Can you work these out from the model? Positions are in its coordinate system, mm. A direction names the side the tool comes from. Round coordinates to 2 decimals unless told otherwise and drop trailing zeros. Write each loop counter-clockwise with the first axis right and the second up, starting at its lowest first coordinate (ties: lowest second). Pieces come first, ordered by that corner, then holes. Notation, with made-up numbers: M -27,59.25 L 17,59.25 A18 cw 17,79.25 Z; hole C 53,67 d5. An arc over 180 degrees is marked long. Answer as a JSON object with one key per item and string values. Group by question number.
1) If we mould it in two halves opening along Z, with no side actions, what happens to faces 1 (the cylindrical face through (-22.316, 9.268, 5.276)), 2 (the flat face through (-15, 17, 4)), 3 (the cylindrical face through (11.353, 19.746, 14.757)), 4 (the cylindrical face through (-22.316, 9.268, 15.276))? For each: +Z half, -Z half, draft (parallel to the pull), parting line (faces both ways), or undercut.
2) Please list where these lines run through material, in increasing order: L1, parallel to X at y = 9.5, z = 3.5; L2, parallel to Y at x = -3.5, z = 17.75; L3, parallel to X at y = 1, z = 11.75. Write a range as [from, to].
3) I'm going to push flat-ended pins straight in: pin 1 Ø4 at (x, z) = (24.5, 9.5) entering from +Y; pin 2 Ø1.5 at (x, z) = (8.5, 3.5) entering from +Y; pin 3 Ø1.5 at (y, z) = (15.5, 15.5) entering from +X; pin 4 Ø3 at (x, z) = (24.315, 15.2) entering from +Y (3 decimals). Where does each tip first touch, or does it pass through?
4) Suppose I cut it at A-A, the plane y = -14. Write out the boundary of the cut face in (x, z), and give its area (3 significant figures).
5) Suppose I cut it at B-B, the plane x = -7.5. Write out the boundary of the cut face in (y, z).
6) On a 3-axis mill with a long thin cutter (end or side, diameter ignored), from which of +Z, -Z, +X, -X, +Y, -Y can I reach the whole of each face in a straight line? I mean faces 5 (the flat face through (-20.15, 13, 10)), 6 (the flat face through (-15, 17, 17)), 7 (the flat face through (20.15, 13, 10)), 8 (the flat face through (27, 9, 3)), 9 (the flat face through (-18, 15.5, 10)). Say none if no direction works.
from build123d import *

# Parameters (mm, degrees)
EXTRUDE_1_DEPTH        = 20
FILLET_1_R             = 1
CUT_EXTRUDE_1_DEPTH    = 20
SKETCH_3_W             = 51.867663345
SKETCH_3_H             = 35.261757523
CUT_EXTRUDE_2_DEPTH    = 3
SKETCH_4_R             = 6
EXTRUDE_2_DEPTH        = 1
SKETCH_5_R             = 5
EXTRUDE_3_DEPTH        = 0.5
SKETCH_6_R             = 1
EXTRUDE_4_DEPTH        = 4
HOLE_WIZARD_M3_1_D     = 2.5
HOLE_WIZARD_M3_1_DEPTH = 7.5
HOLE_WIZARD_M3_1_TIP   = 0.751075774


with BuildPart() as part:
    # 草图1 → 凸台-拉伸1 (new body)
    with BuildSketch(Plane.XY):
        Polygon((20.15, 8), (27, 8), (27, 10.5), (20.15, 10.5), (20.15, 18.5), (-20.15, 18.5), (-20.15, 10.5), (-27, 10.5), (-27, 8), (-20.15, 8), (-20.15, -19), (20.15, -19), align=None)
    extrude(amount=EXTRUDE_1_DEPTH)

    # 圆角1
    fillet_1_edges = [part.edges().sort_by_distance(p)[0] for p in [
        (-27, 9.25, 20),
        (20.15, 14.5, 0),
        (27, 9.25, 0),
        (20.15, -5.5, 0),
        (0, -19, 0),
        (-20.15, -5.5, 0),
        (-27, 9.25, 0),
        (-20.15, 14.5, 0),
        (-20.15, -5.5, 20),
        (0, -19, 20),
        (-20.15, 18.5, 10),
        (20.15, 18.5, 10),
        (20.15, -19, 10),
        (-20.15, -19, 10),
        (20.15, -5.5, 20),
        (27, 9.25, 20),
        (20.15, 14.5, 20),
        (-20.15, 14.5, 20),
    ]]
    fillet(fillet_1_edges, radius=FILLET_1_R)

    # 草图2 → 切除-拉伸1 (cut)
    with BuildSketch(Plane(origin=(0, 10.5, 0), x_dir=(1, 0, 0), z_dir=(0, 1, 0))):
        with BuildLine():
            Line((-26.148030278, -4.4), (-29.222738853, -4.4))
            Line((-29.222738853, -4.4), (-29.222738853, -6))
            Line((-29.222738853, -6), (-26.148030278, -6))
            ThreePointArc((-26.148030278, -6), (-22.315, -5.2), (-26.148030278, -4.4))
        make_face()
        with BuildLine():
            Line((-26.148030278, -14.4), (-29.222738853, -14.4))
            Line((-29.222738853, -14.4), (-29.222738853, -16))
            Line((-29.222738853, -16), (-26.148030278, -16))
            ThreePointArc((-26.148030278, -16), (-22.315, -15.2), (-26.148030278, -14.4))
        make_face()
        with BuildLine():
            Line((26.148030278, -16), (29.222738853, -16))
            Line((29.222738853, -16), (29.222738853, -14.4))
            Line((29.222738853, -14.4), (26.148030278, -14.4))
            ThreePointArc((26.148030278, -14.4), (22.315, -15.2), (26.148030278, -16))
        make_face()
        with BuildLine():
            Line((29.222738853, -4.4), (29.222738853, -6))
            Line((29.222738853, -6), (26.148030278, -6))
            ThreePointArc((26.148030278, -6), (22.315, -5.2), (26.148030278, -4.4))
            Line((26.148030278, -4.4), (29.222738853, -4.4))
        make_face()
    extrude(amount=-CUT_EXTRUDE_1_DEPTH, mode=Mode.SUBTRACT)

    # 草图3 → 切除-拉伸2 (cut)
    with BuildSketch(Plane(origin=(0, 18.5, 0), x_dir=(1, 0, 0), z_dir=(0, 1, 0))):
        with Locations((-0.933831673, -10.85793672)):
            Rectangle(SKETCH_3_W, SKETCH_3_H)
        with BuildLine():
            Line((-14, 0), (8, 0))
            ThreePointArc((8, 0), (18, -10), (8, -20))
            Line((8, -20), (-14, -20))
            ThreePointArc((-14, -20), (-14.707106781, -19.707106781), (-15, -19))
            Line((-15, -19), (-15, -14))
            ThreePointArc((-15, -14), (-17, -10), (-15, -6))
            Line((-15, -6), (-15, -1))
            ThreePointArc((-15, -1), (-14.707106781, -0.292893219), (-14, 0))
        make_face(mode=Mode.SUBTRACT)
    extrude(amount=-CUT_EXTRUDE_2_DEPTH, mode=Mode.SUBTRACT)

    # 草图4 → 凸台-拉伸2 (add)
    with BuildSketch(Plane(origin=(0, 18.5, 0), x_dir=(1, 0, 0), z_dir=(0, 1, 0))):
        with Locations((9.85, -10)):
            Circle(SKETCH_4_R)
    extrude(amount=EXTRUDE_2_DEPTH)

    # 草图5 → 凸台-拉伸3 (add)
    with BuildSketch(Plane(origin=(0, 19.5, 0), x_dir=(1, 0, 0), z_dir=(0, 1, 0))):
        with Locations(Location((9.851314919, -9.987632383, 0), (0, 0, 270))):
            Circle(SKETCH_5_R)
    extrude(amount=EXTRUDE_3_DEPTH)

    # 草图6 → 凸台-拉伸4 (add)
    with BuildSketch(Plane(origin=(0, 20, 0), x_dir=(1, 0, 0), z_dir=(0, 1, 0))):
        with BuildLine():
            Line((10.284120444, -7.537980617), (10.353579715, -7.144057516))
            ThreePointArc((10.353579715, -7.144057516), (9.85, -7.1), (9.346420285, -7.144057516))
            Line((9.346420285, -7.144057516), (9.415879556, -7.537980617))
            ThreePointArc((9.415879556, -7.537980617), (8.994949642, -7.650768448), (8.6, -7.834936491))
            Line((8.6, -7.834936491), (8.4, -7.488526329))
            ThreePointArc((8.4, -7.488526329), (7.985915932, -7.778471115), (7.628471115, -8.135915932))
            Line((7.628471115, -8.135915932), (7.934888892, -8.393030976))
            ThreePointArc((7.934888892, -8.393030976), (7.684936491, -8.75), (7.500768448, -9.144949642))
            Line((7.500768448, -9.144949642), (7.1248914, -9.008141584))
            ThreePointArc((7.1248914, -9.008141584), (6.994057516, -9.496420285), (6.95, -10))
            Line((6.95, -10), (7.35, -10))
            ThreePointArc((7.35, -10), (7.387980617, -10.434120444), (7.500768448, -10.855050358))
            Line((7.500768448, -10.855050358), (7.1248914, -10.991858416))
            ThreePointArc((7.1248914, -10.991858416), (7.338526329, -11.45), (7.628471115, -11.864084068))
            Line((7.628471115, -11.864084068), (7.934888892, -11.606969024))
            ThreePointArc((7.934888892, -11.606969024), (8.243030976, -11.915111108), (8.6, -12.165063509))
            Line((8.6, -12.165063509), (8.4, -12.511473671))
            ThreePointArc((8.4, -12.511473671), (8.858141584, -12.7251086), (9.346420285, -12.855942484))
            Line((9.346420285, -12.855942484), (9.415879556, -12.462019383))
            ThreePointArc((9.415879556, -12.462019383), (9.85, -12.5), (10.284120444, -12.462019383))
            Line((10.284120444, -12.462019383), (10.353579715, -12.855942484))
            ThreePointArc((10.353579715, -12.855942484), (10.841858416, -12.7251086), (11.3, -12.511473671))
            Line((11.3, -12.511473671), (11.1, -12.165063509))
            ThreePointArc((11.1, -12.165063509), (11.456969024, -11.915111108), (11.765111108, -11.606969024))
            Line((11.765111108, -11.606969024), (12.071528885, -11.864084068))
            ThreePointArc((12.071528885, -11.864084068), (12.361473671, -11.45), (12.5751086, -10.991858416))
            Line((12.5751086, -10.991858416), (12.199231552, -10.855050358))
            ThreePointArc((12.199231552, -10.855050358), (12.312019383, -10.434120444), (12.35, -10))
            Line((12.35, -10), (12.75, -10))
            ThreePointArc((12.75, -10), (12.705942484, -9.496420285), (12.5751086, -9.008141584))
            Line((12.5751086, -9.008141584), (12.199231552, -9.144949642))
            ThreePointArc((12.199231552, -9.144949642), (12.015063509, -8.75), (11.765111108, -8.393030976))
            Line((11.765111108, -8.393030976), (12.071528885, -8.135915932))
            ThreePointArc((12.071528885, -8.135915932), (11.714084068, -7.778471115), (11.3, -7.488526329))
            Line((11.3, -7.488526329), (11.1, -7.834936491))
            ThreePointArc((11.1, -7.834936491), (10.705050358, -7.650768448), (10.284120444, -7.537980617))
        make_face()
        with Locations(Location((9.85, -10, 0), (0, 0, 270))):
            Circle(SKETCH_6_R, mode=Mode.SUBTRACT)
    extrude(amount=EXTRUDE_4_DEPTH)

    # M3 螺纹孔1
    with Locations(Plane(origin=(9.85, 24, 10), x_dir=(0, 0, 1), z_dir=(0, 1, 0))):
        with Locations((0, 0)):
            Hole(HOLE_WIZARD_M3_1_D / 2, depth=HOLE_WIZARD_M3_1_DEPTH)
            with Locations((0, 0, -(HOLE_WIZARD_M3_1_DEPTH + HOLE_WIZARD_M3_1_TIP / 2))):  # 118° drill point
                Cone(0, HOLE_WIZARD_M3_1_D / 2, HOLE_WIZARD_M3_1_TIP, mode=Mode.SUBTRACT)


solid = part.part
Results:
{
 "1": {"face 1": "undercut", "face 2": "draft", "face 3": "parting line", "face 4": "undercut"},
 "2": {"L1": "[-27, -25.37], [-23.26, 23.26], [25.37, 27]", "L2": "[-19, 18.5]", "L3": "[-20.15, 20.15]"},
 "3": {"pin 1": "y = 10.5", "pin 2": "y = 19.5", "pin 3": "x = 20.15", "pin 4": "through"},
 "4": {"outline": "M -20.15,1 A1 ccw -19.15,0 L 19.15,0 A1 ccw 20.15,1 L 20.15,19 A1 ccw 19.15,20 L -19.15,20 A1 ccw -20.15,19 Z", "area": "805 mm^2"},
 "5": {"outline": "M -19,1 A1 ccw -18,0 L 18.5,0 L 18.5,20 L -18,20 A1 ccw -19,19 Z"},
 "6": {"face 5": "+Z, -Z, -X, +Y", "face 6": "+Z, -X, +Y", "face 7": "+Z, -Z, +X, +Y", "face 8": "+Z, -Z, +X, +Y, -Y", "face 9": "-X, +Y"}
}
